```python
from build123d import *

# Parameters (mm, degrees)
BASPROSKE_W         = 4
BASPROSKE_H         = 7.875
TOOTHCUT_DEPTH      = 12.833480046
TEETHCUTS_COUNT     = 12
TEETHCUTS_ANGLE     = 330
BORSKE_R            = 3.625
BORE_DEPTH          = 50.0000508
SKETCH1_R           = 4.5
SKETCH1_R_2         = 3.5
BOSS_EXTRUDE1_DEPTH = 1
CUT_EXTRUDE2_DEPTH  = 2


with BuildPart() as part:
    # BasProSke → Base-Revolve (revolve)
    with BuildSketch(Plane(origin=(0, 0, 0), x_dir=(1, 0, 0), z_dir=(0, 1, 0)), mode=Mode.PRIVATE) as base_revolve_sk:
        with Locations((2, 3.9375)):
            Rectangle(BASPROSKE_W, BASPROSKE_H)
    revolve(base_revolve_sk.sketch.rotate(Axis((-10, 0, 0), (1, 0, 0)), 180), axis=Axis((-10, 0, 0), (1, 0, 0)))

    # TooCutSke → ToothCut (cut, through all)
    with BuildSketch(Plane(origin=(0, 0, 0), x_dir=(0, 0, -1), z_dir=(1, 0, 0))):
        with BuildLine():
            ThreePointArc((0.631439839, 5.305305014), (0, 5.34275), (-0.631439839, 5.305305014))
            ThreePointArc((-0.631439839, 5.305305014), (-0.93992237, 6.654932089), (-1.876748184, 7.674251521))
            ThreePointArc((-1.876748184, 7.674251521), (0, 7.9004), (1.876748184, 7.674251521))
            ThreePointArc((1.876748184, 7.674251521), (0.93992237, 6.654932089), (0.631439839, 5.305305014))
        make_face()
    toothcut = extrude(amount=TOOTHCUT_DEPTH, mode=Mode.SUBTRACT)

    # TeethCuts: ToothCut ×12 about axis
    teethcuts_axis = Axis((-10, 0, 0), (1, 0, 0))
    for i in range(1, TEETHCUTS_COUNT):
        add(toothcut.rotate(teethcuts_axis, i * TEETHCUTS_ANGLE / (TEETHCUTS_COUNT - 1)), mode=Mode.SUBTRACT)

    # BorSke → Bore (cut, symmetric)
    with BuildSketch(Plane(origin=(0, 0, 0), x_dir=(0, 0, -1), z_dir=(1, 0, 0))):
        with Locations(Location((0, 0, 0), (0, 0, 180))):
            Circle(BORSKE_R)
    extrude(amount=BORE_DEPTH, both=True, mode=Mode.SUBTRACT)

    # Sketch1 → Boss-Extrude1 (add)
    with BuildSketch(Plane.ZY):
        with Locations(Location((0, 0, 0), (0, 0, 180))):
            Circle(SKETCH1_R)
        Circle(SKETCH1_R_2, mode=Mode.SUBTRACT)
    extrude(amount=BOSS_EXTRUDE1_DEPTH)

    # Sketch3 → Cut-Extrude2 (cut)
    with BuildSketch(Plane(origin=(4, 0, 0), x_dir=(0, 0, -1), z_dir=(1, 0, 0))):
        with BuildLine():
            Line((0.328125, 3.484585195), (16.1875, 1.99119154))
            ThreePointArc((16.1875, 1.99119154), (18, 0), (16.1875, -1.99119154))
            Line((16.1875, -1.99119154), (0.328125, -3.484585195))
            ThreePointArc((0.328125, -3.484585195), (-3.5, 0), (0.328125, 3.484585195))
        make_face()
    extrude(amount=-CUT_EXTRUDE2_DEPTH, mode=Mode.SUBTRACT)


solid = part.part
```
Source: CAD feature listing. Evaluate the final solid. Frame: model axes, mm. A direction names the side the tool comes from. Coordinates: 2 decimals unless noted, no trailing zeros. Write each loop counter-clockwise with the first axis right and the second up, starting at its lowest first coordinate (ties: lowest second). Pieces come first, ordered by that corner, then holes. Notation, with made-up numbers: (-4.75, 18) - (2.25, 18) arc R25 cw to (2.25, 31) - close; hole circle Ø7 at (-35.5, 78). An arc over 180 degrees is marked (long way). Answer as a JSON object with one key per item and string values.
Q1. Draft query along Z for faces 4 (the cylindrical face through (1.972, -4.11, 5.273)), 5 (the flat face through (0, 0, -5)), 6 (the cylindrical face through (1.97, 6.62, 0.92)), 7 (the cylindrical face through (1.972, 4.631, 2.664)). Return one class per face: released by +Z, released by -Z, zero draft, split by the parting line, or undercut.
Ans:
{"face 4": "released by +Z", "face 5": "zero draft", "face 6": "undercut", "face 7": "undercut"}
Q2. Section query D-D, the plane z = -2.75. Output: boundary loops of the cut face in (x, y), plus the area to 3 significant figures.
Ans:
{"outline": "(-1, -3.56) - (0, -3.56) - (0, -4.58) - (4, -4.58) - (4, -3.26) - (2, -3.26) - (2, -2.36) - (0, -2.36) - (0, -2.17) - (-1, -2.17) - close; (-1, 2.17) - (0, 2.17) - (0, 2.36) - (2, 2.36) - (2, 3.26) - (4, 3.26) - (4, 4.58) - (0, 4.58) - (0, 3.56) - (-1, 3.56) - close", "area": "17.0 mm2"}
Q3. Set-up query: faces 1 (the cylindrical face through (-0.49, -3.04, 3.32)), 2 (the cylindrical face through (1.972, -2.514, 6.235)), 3 (the flat face through (3.01, -3.25, -2.83)). Return all of +Z, -Z, +X, -X, +Y, -Y with unobstructed straight access to the full face (end or side cutting, diameter ignored); none if empty.
Ans:
{"face 1": "-X", "face 2": "+X, -X", "face 3": "+X"}
Q4. Section query C-C, the plane x = -0.3. Output: boundary loops of the cut face in (y, z), plus the area to 3 significant figures.
Ans:
{"outline": "circle Ø9 at (0, 0); hole circle Ø7 at (0, 0)", "area": "25.1 mm2"}
Q5. Material intervals for line 1 (Y direction, x = 2, z = 0) (3 decimals); line 2 (Y direction, x = -0.8, z = 0); line 3 (Z direction, x = 3.3, y = 4.75), sorted ascending. Write a range as [from, to].
Ans:
{"line 1": "y = [-5.343, -3.625], [3.625, 5.343]", "line 2": "y = [-4.5, -3.5], [3.5, 4.5]", "line 3": "z = [-5.58, -3.52], [-2.45, 2.45], [3.52, 5.58]"}
Q6. First-contact query: pin 1 Ø9 at (y, z) = (0, 0) entering from +X; pin 2 Ø1.9 at (y, z) = (-1, -4) entering from +X. Flat tips, straight axial feed; report the tip coordinate or a pass-through.
Ans:
{"pin 1": "stops at x = 4", "pin 2": "stops at x = 2"}
Q7. Section query A-A, the plane y = 0. Output: boundary loops of the cut face in (x, z) (3 decimals), plus the area to 3 significant figures.
Ans:
{"outline": "(-1, -4.5) - (0, -4.5) - (0, -5.343) - (2, -5.343) - (2, -3.625) - (0, -3.625) - (0, -3.5) - (-1, -3.5) - close; (-1, 3.5) - (0, 3.5) - (0, 3.625) - (4, 3.625) - (4, 5.343) - (0, 5.343) - (0, 4.5) - (-1, 4.5) - close", "area": "12.3 mm2"}
Q8. Section query B-B, the plane z = 0. Output: boundary loops of the cut face in (x, y) (3 decimals), plus the area to 3 significant figures.
Ans:
{"outline": "(-1, -4.5) - (0, -4.5) - (0, -5.343) - (4, -5.343) - (4, -3.625) - (0, -3.625) - (0, -3.5) - (-1, -3.5) - close; (-1, 3.5) - (0, 3.5) - (0, 3.625) - (4, 3.625) - (4, 5.343) - (0, 5.343) - (0, 4.5) - (-1, 4.5) - close", "area": "15.7 mm2"}
